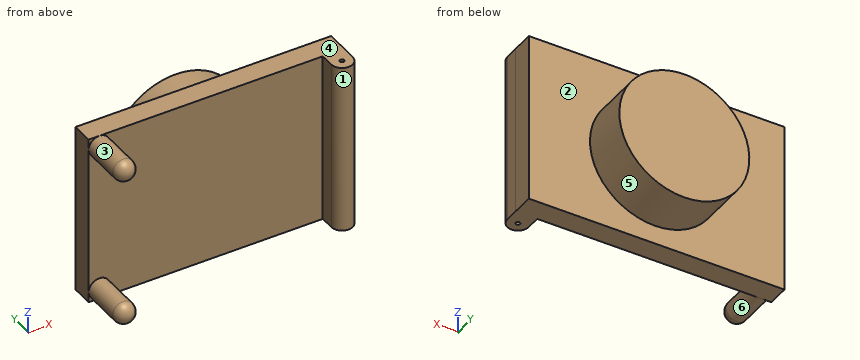
from build123d import *

# Parameters (mm, degrees)
SKETCH1_W           = 301
SKETCH1_H           = 202
BOSS_EXTRUDE1_DEPTH = 60
CUT_EXTRUDE1_DEPTH  = 259.948353924
SKETCH5_R           = 12.5
BOSS_EXTRUDE2_DEPTH = 59.1
FILLET1_R           = 12.5
SKETCH2_R           = 2.5
CUT_EXTRUDE2_DEPTH  = 259.948353924
SKETCH6_R           = 76.5
BOSS_EXTRUDE3_DEPTH = 57


with BuildPart() as part:
    # Sketch1 → Boss-Extrude1 (new body)
    with BuildSketch(Plane(origin=(0, 0, 0), x_dir=(1, 0, 0), z_dir=(0, 1, 0))):
        Rectangle(SKETCH1_W, SKETCH1_H)
    extrude(amount=BOSS_EXTRUDE1_DEPTH)

    # Sketch4 → Cut-Extrude1 (cut, through all)
    with BuildSketch(Plane.XY.offset(101)):
        with BuildLine():
            Line((125.3, 18), (125.1, 34.6))
            Line((125.1, 34.6), (-150.5, 34.6))
            Line((-150.5, 34.6), (-150.5, 0))
            Line((-150.5, 0), (150.5, 0))
            Line((150.5, 0), (150.5, 34.6))
            Line((150.5, 34.6), (150.3, 18))
            ThreePointArc((150.3, 18), (137.8, 5.5), (125.3, 18))
        make_face()
    extrude(amount=-CUT_EXTRUDE1_DEPTH, mode=Mode.SUBTRACT)

    # Sketch5 → Boss-Extrude2 (add)
    with BuildSketch(Plane.XZ.offset(-34.6)):
        with Locations(Location((-138, 88.5, 0), (0, 0, 90))):
            Circle(SKETCH5_R)
        with Locations(Location((-138, -88.5, 0), (0, 0, 270))):
            Circle(SKETCH5_R)
    extrude(amount=BOSS_EXTRUDE2_DEPTH)

    # Fillet1
    fillet1_edges = [part.edges().sort_by_distance(p)[0] for p in [
        (-138, -24.5, 76),
        (-138, -24.5, -76),
    ]]
    fillet(fillet1_edges, radius=FILLET1_R)

    # Sketch2 → Cut-Extrude2 (cut, through all)
    with BuildSketch(Plane.XY.offset(101)):
        with Locations((137.8, 18)):
            Circle(SKETCH2_R)
    extrude(amount=-CUT_EXTRUDE2_DEPTH, mode=Mode.SUBTRACT)

    # Sketch6 → Boss-Extrude3 (add)
    with BuildSketch(Plane(origin=(0, 60, 0), x_dir=(1, 0, 0), z_dir=(0, 1, 0))):
        with Locations(Location((2, 2.5, 0), (0, 0, 90))):
            Circle(SKETCH6_R)
    extrude(amount=BOSS_EXTRUDE3_DEPTH)


solid = part.part
Geometry: final body of the model. Coordinates: model frame, mm. Face numbers are marked on the shaded views. A direction names the side the tool comes from. Round coordinates to 2 decimals unless told otherwise and drop trailing zeros. Order: outer loops, then holes, each group sorted by start corner. A loop starts at its lowest first (then second) coordinate and runs counter-clockwise, first axis right, second up.
Q1. Section C-C, the plane x = 2. Output: boundary loops of the cut face in (y, z).
Result sheet:
outline: (34.6, -101) - (60, -101) - (60, -79) - (117, -79) - (117, 74) - (60, 74) - (60, 101) - (34.6, 101) - close
Q2. Mould query, pull axis X, two halves, no side actions, for the marked faces 4, 5 and 6. Classes: released by +X, released by -X, zero draft, split by the parting line, or undercut.
Result sheet:
face 4: zero draft
face 5: split by the parting line
face 6: undercut
Q3. Material intervals for probe 1 along Y at (x, z) = (137.8, -9.5); probe 2 along Y at (x, z) = (-16, 6); probe 3 along Y at (x, z) = (81, 86), sorted ascending.
Result sheet:
probe 1: y = 5.5 to 15.5, 20.5 to 60
probe 2: y = 34.6 to 117
probe 3: y = 34.6 to 60
Q4. Section A-A, the plane z = -44.5. Output: boundary loops of the cut face in (x, y).
Result sheet:
outline: (-150.5, 34.6) - (125.1, 34.6) - (125.3, 18) arc R12.5 ccw to (150.3, 18) - (150.5, 34.6) - (150.5, 60) - (65.94, 60) - (65.94, 117) - (-61.94, 117) - (-61.94, 60) - (-150.5, 60) - close; hole circle Ø5 at (137.8, 18)
Q5. Section B-B, the plane y = 10.5. Output: boundary loops of the cut face in (x, z), and give its area (3 significant figures).
Result sheet:
outline: circle Ø25 at (-138, -88.5); circle Ø25 at (-138, 88.5); (127.8, -101) - (147.8, -101) - (147.8, 101) - (127.8, 101) - close
area: 5,020 mm2
Q6. Access query for the marked faces 1, 2 and 3. Directions: +Z, -Z, +X, -X, +Y, -Y. A direction counts if a zero-diameter tool reaches every point of the face in a straight line with its end or side. Return the directions, or none.
Result sheet:
face 1: +Z, -Z, -Y
face 2: +Y
face 3: -Y
Q7. Section D-D, the plane y = 82. Output: boundary loops of the cut face in (x, z).
Result sheet:
outline: circle Ø153 at (2, -2.5)
Q8. Pin query (flat end, axial travel): pin 1 (3.5 mm diameter, centred on x = -147, z = -94.5, fed in from -Y) (3 decimals); pin 2 (4 mm diameter, centred on x = -2, z = 14, fed in from -Y); pin 3 (3 mm diameter, centred on x = 137.8, y = 18, fed in from +Z); pin 4 (10 mm diameter, centred on y = 18, z = 72.5, fed in from -X). Return the tip coordinate at first contact, or that it passes through.
Result sheet:
pin 1: stops at y = -20.605
pin 2: stops at y = 34.6
pin 3: passes through
pin 4: stops at x = -143.94
